For this review, take the finished solid that the model builds, in its own axes (mm). Face numbers are marked on the shaded views. A direction names the side the tool comes from. Give positions to 0.01 mm unless a question says otherwise; leave off trailing zeros. Loops run counter-clockwise (first coordinate to the right, second up) from the corner with the lowest first, then second, coordinate; pieces in that order, holes last. Notation, with made-up numbers: (-17.75, 18) - (4.25, 18) arc R22 ccw to (4.25, 34) - close; hole circle Ø5 at (80, 2.25). An arc over 180 degrees is marked (long way). Answer in a Markdown table with one row per item.
```python
from build123d import *

# Parameters (mm, degrees)
SKETCH1_R           = 1.5
SKETCH1_W           = 11.811
SKETCH1_H           = 11.811
BOSS_EXTRUDE1_DEPTH = 5.9944


with BuildPart() as part:
    # Sketch1 → Boss-Extrude1 (new body)
    with BuildSketch(Plane.XY):
        Polygon((44.45, -60.325), (50.4444, -60.325), (50.4444, -15.875), (44.45, -15.875), (44.45, 0), (36.603489481, 0), (36.603489481, 5.9944), (11.203489481, 5.9944), (11.203489481, 0), (0, 0), (0, -76.2), (44.45, -76.2), align=None)
        with Locations(Location((6.595000018, -67.199999966, 0), (0, 0, 180))):
            Circle(SKETCH1_R, mode=Mode.SUBTRACT)
        with Locations(Location((37.854999982, -67.199999966, 0), (0, 0, 180))):
            Circle(SKETCH1_R, mode=Mode.SUBTRACT)
        with Locations((22.225, -68.2625)):
            Rectangle(SKETCH1_W, SKETCH1_H, mode=Mode.SUBTRACT)
    extrude(amount=BOSS_EXTRUDE1_DEPTH)


solid = part.part
```
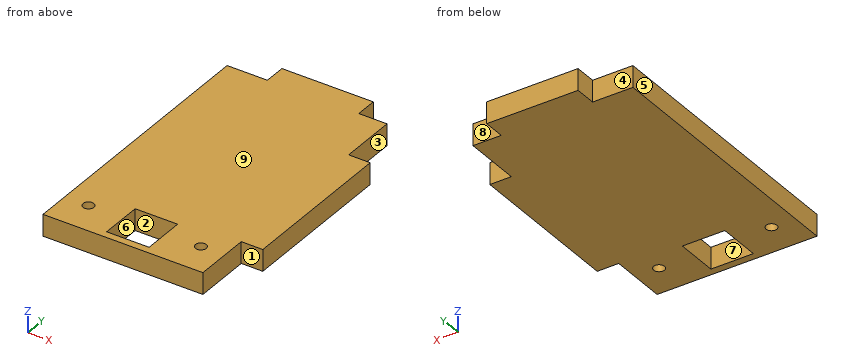
1. Mouldability with a two-part tool opening along Y and no side actions: class the marked faces 6, 7, 8 and 9 as released by +Y, released by -Y, zero draft, split by the parting line, or undercut.
Values:
| item | result |
|---|---|
| face 6 | undercut |
| face 7 | undercut |
| face 8 | released by +Y |
| face 9 | zero draft |
2. Clearance check with flat-ended pins moving along their axes: pin 1 (1.8 mm diameter, centred on y = -70.5, z = 4.5, fed in from +X); pin 2 (3 mm diameter, centred on x = 47.5, z = 4, fed in from -Y) (3 decimals); pin 3 (3 mm diameter, centred on x = 40, z = 4, fed in from +Y); pin 4 (1.8 mm diameter, centred on x = 6.595, y = -67.2, fed in from -Z). State where each tip first meets the part, or that it passes through.
Values:
| item | result |
|---|---|
| pin 1 | stops at x = 44.45 |
| pin 2 | stops at y = -60.325 |
| pin 3 | stops at y = 0 |
| pin 4 | passes through |
3. We need section D-D, the plane x = 9. Give the boundary of the cut face in (y, z).
Values:
| item | result |
|---|---|
| outline | (-76.2, 0) - (0, 0) - (0, 5.99) - (-76.2, 5.99) - close |
4. Wall thickness on line 1 (Y direction, x = 38, z = 2.2); line 2 (Y direction, x = 16.5, z = 1.1); line 3 (X direction, y = -71, z = 3.9): over which ranges is each line inside the solid? List them lowest first. Write a range as [from, to].
Values:
| item | result |
|---|---|
| line 1 | y = [-76.2, -68.69], [-65.71, 0] |
| line 2 | y = [-76.2, -74.17], [-62.36, 5.99] |
| line 3 | x = [0, 16.32], [28.13, 44.45] |
5. For the marked faces 1, 2, 3, 4 and 5, list the 3-axis set-ups (+Z, -Z, +X, -X, +Y, -Y) from which the entire face can be reached by the end or side of a thin tool; tool diameter is ignored.
Values:
| item | result |
|---|---|
| face 1 | +Z, -Z, +X, -Y |
| face 2 | +Z, -Z |
| face 3 | +Z, -Z, +X, +Y |
| face 4 | +Z, -Z, -X, +Y |
| face 5 | +Z, -Z, -X, +Y, -Y |
6. We need section A-A, the plane x = 17.5. Give the boundary of the cut face in (y, z), and give its area (3 significant figures).
Values:
| item | result |
|---|---|
| outline | (-76.2, 0) - (-74.17, 0) - (-74.17, 5.99) - (-76.2, 5.99) - close; (-62.36, 0) - (5.99, 0) - (5.99, 5.99) - (-62.36, 5.99) - close |
| area | 422 mm^2 |
7. We need section B-B, the plane y = -67.2. Count the separate pieces of the cut face and the enclosed holes in it, and give its area (3 significant figures).
Values:
| item | result |
|---|---|
| separate pieces | 4 |
| enclosed holes | 0 |
| area | 160 mm^2 |
